```python
from build123d import *

# Parameters (mm, degrees)
SKETCH_1_W                         = 397
SKETCH_1_H                         = 497
SKETCH_1_W_2                       = 22.1
SKETCH_1_H_2                       = 22.1
SM_BASE_FLANGE_1_DEPTH             = 2
SM_EDGE_FLANGE_1_STRIP_W           = 8.6
SM_EDGE_FLANGE_1_STRIP_H           = 2
SM_EDGE_FLANGE_1_STRIP_CUT_DEPTH   = 497
SM_EDGE_FLANGE_1_STRIP_2_W         = 8.6
SM_EDGE_FLANGE_1_STRIP_2_H         = 2
SM_EDGE_FLANGE_1_STRIP_CUT_2_DEPTH = 497
SM_EDGE_FLANGE_1_DEPTH             = 497
SM_EDGE_FLANGE_1_BEND_DEPTH        = 497
SM_START                           = -198.5
SM_EDGE_FLANGE_2_DEPTH             = 397
SM_EDGE_FLANGE_2_2_DEPTH           = 2.3
SM_START_2                         = 196.2
SM_EDGE_FLANGE_2_3_DEPTH           = 2.3
SM_START_3                         = -196.2
SM_EDGE_FLANGE_2_4_DEPTH           = 392.4
SKETCH_18_R                        = 1.6
CUT_EXTRUDE_1_DEPTH                = 10


# Read off the part's stored shape, not the designer's step: 边线-法兰2
# Sheet-metal steps are written as plain solids
with BuildPart() as part:
    # Sketch 1 → 基体-法兰1 (new body)
    with BuildSketch(Plane.XY):
        Rectangle(SKETCH_1_W, SKETCH_1_H)
        with Locations((-146.5, 0)):
            Rectangle(SKETCH_1_W_2, SKETCH_1_H_2, mode=Mode.SUBTRACT)
    extrude(amount=-SM_BASE_FLANGE_1_DEPTH)

    # 边线-法兰1 strip (across the edge) → 边线-法兰1 strip cut (cut)
    with BuildSketch(Plane(origin=(198.5, 248.5, -2), x_dir=(-1, 0, 0), z_dir=(0, -1, 0))):
        with Locations((-2, -1)):
            Rectangle(SM_EDGE_FLANGE_1_STRIP_W, SM_EDGE_FLANGE_1_STRIP_H)
    extrude(amount=SM_EDGE_FLANGE_1_STRIP_CUT_DEPTH, mode=Mode.SUBTRACT)

    # 边线-法兰1 strip 2 (across the edge) → 边线-法兰1 strip cut 2 (cut)
    with BuildSketch(Plane(origin=(-198.5, -248.5, -2), x_dir=(1, 0, 0), z_dir=(0, 1, 0))):
        with Locations((-2, -1)):
            Rectangle(SM_EDGE_FLANGE_1_STRIP_2_W, SM_EDGE_FLANGE_1_STRIP_2_H)
    extrude(amount=SM_EDGE_FLANGE_1_STRIP_CUT_2_DEPTH, mode=Mode.SUBTRACT)

    # 边线-法兰1 section (across the edge) → 边线-法兰1 (add)
    with BuildSketch(Plane(origin=(198.5, 248.5, -2), x_dir=(-1, 0, 0), z_dir=(0, -1, 0))):
        with BuildLine():
            Line((0, 0.3), (0, 13))
            Line((0, 13), (2, 13))
            Line((2, 13), (2, 0.3))
            ThreePointArc((2, 0.3), (2.087867966, 0.087867966), (2.3, 0))
            Line((2.3, 0), (2.3, -2))
            ThreePointArc((2.3, -2), (0.673654403, -1.326345597), (0, 0.3))
        make_face()
    extrude(amount=SM_EDGE_FLANGE_1_DEPTH)

    # 边线-法兰1 section 2 (across the edge) → 边线-法兰1 bend (add)
    with BuildSketch(Plane(origin=(-198.5, -248.5, -2), x_dir=(1, 0, 0), z_dir=(0, 1, 0))):
        with BuildLine():
            Line((0, 0.3), (0, 13))
            Line((0, 13), (2, 13))
            Line((2, 13), (2, 0.3))
            ThreePointArc((2, 0.3), (2.087867966, 0.087867966), (2.3, 0))
            Line((2.3, 0), (2.3, -2))
            ThreePointArc((2.3, -2), (0.673654403, -1.326345597), (0, 0.3))
        make_face()
    extrude(amount=SM_EDGE_FLANGE_1_BEND_DEPTH)

    # 边线-法兰2 outline → 边线-法兰2 (cut)
    with BuildSketch(Plane.YZ.offset(SM_START)):
        with BuildLine():
            Line((-246.5, -2.3), (-246.2, -2.3))
            Line((-246.2, -2.3), (-246.2, -2))
            ThreePointArc((-246.2, -2), (-246.412132034, -2.087867966), (-246.5, -2.3))
        make_face()
        with BuildLine():
            ThreePointArc((-248.5, -2.3), (-247.826345597, -0.673654403), (-246.2, 0))
            Line((-246.2, 0), (-248.5, 0))
            Line((-248.5, 0), (-248.5, -2.3))
        make_face()
        with BuildLine():
            ThreePointArc((246.5, -2.3), (246.412132034, -2.087867966), (246.2, -2))
            Line((246.2, -2), (246.2, -2.3))
            Line((246.2, -2.3), (246.5, -2.3))
        make_face()
        with BuildLine():
            Line((248.5, 0), (246.2, 0))
            ThreePointArc((246.2, 0), (247.826345597, -0.673654403), (248.5, -2.3))
            Line((248.5, -2.3), (248.5, 0))
        make_face()
    extrude(amount=SM_EDGE_FLANGE_2_DEPTH, mode=Mode.SUBTRACT)

    # Sm Edge Flange 2 2 outline → Sm Edge Flange 2 2 (cut)
    with BuildSketch(Plane.YZ.offset(SM_START)):
        with BuildLine():
            Line((-248.5, -2.3), (-246.5, -2.3))
            ThreePointArc((-246.5, -2.3), (-246.412132034, -2.087867966), (-246.2, -2))
            Line((-246.2, -2), (-246.2, 0))
            ThreePointArc((-246.2, 0), (-247.826345597, -0.673654403), (-248.5, -2.3))
        make_face()
        with BuildLine():
            ThreePointArc((248.5, -2.3), (247.826345597, -0.673654403), (246.2, 0))
            Line((246.2, 0), (246.2, -2))
            ThreePointArc((246.2, -2), (246.412132034, -2.087867966), (246.5, -2.3))
            Line((246.5, -2.3), (248.5, -2.3))
        make_face()
    extrude(amount=SM_EDGE_FLANGE_2_2_DEPTH, mode=Mode.SUBTRACT)

    # Sm Edge Flange 2 3 outline → Sm Edge Flange 2 3 (cut)
    with BuildSketch(Plane.YZ.offset(SM_START_2)):
        with BuildLine():
            Line((-248.5, -2.3), (-246.5, -2.3))
            ThreePointArc((-246.5, -2.3), (-246.412132034, -2.087867966), (-246.2, -2))
            Line((-246.2, -2), (-246.2, 0))
            ThreePointArc((-246.2, 0), (-247.826345597, -0.673654403), (-248.5, -2.3))
        make_face()
        with BuildLine():
            ThreePointArc((248.5, -2.3), (247.826345597, -0.673654403), (246.2, 0))
            Line((246.2, 0), (246.2, -2))
            ThreePointArc((246.2, -2), (246.412132034, -2.087867966), (246.5, -2.3))
            Line((246.5, -2.3), (248.5, -2.3))
        make_face()
    extrude(amount=SM_EDGE_FLANGE_2_3_DEPTH, mode=Mode.SUBTRACT)

    # Sm Edge Flange 2 4 outline → Sm Edge Flange 2 4 (add)
    with BuildSketch(Plane.YZ.offset(SM_START_3)):
        with BuildLine():
            Line((-246.5, -15), (-246.5, -2.3))
            ThreePointArc((-246.5, -2.3), (-246.412132034, -2.087867966), (-246.2, -2))
            Line((-246.2, -2), (-248.48035085, -2))
            ThreePointArc((-248.48035085, -2), (-248.495082456, -2.149678603), (-248.5, -2.3))
            Line((-248.5, -2.3), (-248.5, -15))
            Line((-248.5, -15), (-246.5, -15))
        make_face()
        with BuildLine():
            Line((248.48035085, -2), (246.2, -2))
            ThreePointArc((246.2, -2), (246.412132034, -2.087867966), (246.5, -2.3))
            Line((246.5, -2.3), (246.5, -15))
            Line((246.5, -15), (248.5, -15))
            Line((248.5, -15), (248.5, -2.3))
            ThreePointArc((248.5, -2.3), (248.495082456, -2.149678603), (248.48035085, -2))
        make_face()
    extrude(amount=SM_EDGE_FLANGE_2_4_DEPTH)

    # 草图18 → 切除-拉伸1 (cut)
    with BuildSketch(Plane(origin=(198.5, 0, 0), x_dir=(0, 0, -1), z_dir=(1, 0, 0))):
        with Locations((5.5, -183.25)):
            Circle(SKETCH_18_R)
        with Locations((12.5, -183.25)):
            Circle(SKETCH_18_R)
        with Locations((5.5, -168.75)):
            Circle(SKETCH_18_R)
        with Locations((12.5, -168.75)):
            Circle(SKETCH_18_R)
        with Locations(Location((12.5, 168.75, 0), (0, 0, 180))):
            Circle(SKETCH_18_R)
        with Locations(Location((5.5, 168.75, 0), (0, 0, 180))):
            Circle(SKETCH_18_R)
        with Locations(Location((12.5, 183.25, 0), (0, 0, 180))):
            Circle(SKETCH_18_R)
        with Locations(Location((5.5, 183.25, 0), (0, 0, 180))):
            Circle(SKETCH_18_R)
    extrude(amount=-CUT_EXTRUDE_1_DEPTH, mode=Mode.SUBTRACT)


solid = part.part
```
The model under review builds one solid part; all positions refer to its coordinate system, in mm. A direction names the side the tool comes from. Coordinates: 2 decimals unless noted, no trailing zeros. Order: outer loops, then holes, each group sorted by start corner. A loop starts at its lowest first (then second) coordinate and runs counter-clockwise, first axis right, second up. Notation, with made-up numbers: (-35, 35.25) -> (-1, 35.25) arc R26 ccw to (-1, 70.25) -> close; hole circle Ø1 at (-20, 26). An arc over 180 degrees is marked (long way). Answer in a Markdown table with one row per item. Add a question column.
Item 1: We need section B-B on x = -171. Write out the cut boundary in (y, z), plus the area to 3 significant figures.
Item 2: To check wall thickness, follow probe 1 along Y at (x, z) = (197.55, -12.5); probe 2 along Y at (x, z) = (26, -2.25); probe 3 along X at (y, z) = (103.5, -3.5). State the ranges of each line that lie inside material, in increasing order.
Item 3: Machinability: for faces 1 (the flat face through (198.5, 3, -9)), 2 (the flat face through (-3, -246.5, -9)), which of the approach directions +Z, -Z, +X, -X, +Y, -Y give a long, thin tool a straight path to every point of the face, cutting with its end or side? Answer none if there is none.
Item 4: Mouldability with a two-part tool opening along Y and no side actions: class faces 3 (the flat face through (-3, 3, -2)), 4 (the flat face through (-3, 246.5, -9)), 5 (the flat face through (-3, 3, 0)), 6 (the flat face through (-3, -248.5, -9)) as +Y half, -Y half, draft (parallel to the pull), parting line (faces both ways), or undercut.
Item 5: We need section A-A on y = 122.5. Write out the cut boundary in (x, z).
Item 6: Clearance check with flat-ended pins moving along their axes: pin 1 (1 mm diameter, centred on x = 197.5, y = 247, fed in from +Z); pin 2 (2.5 mm diameter, centred on x = 197, z = -1, fed in from +Y); pin 3 (1 mm diameter, centred on x = -141.5, z = -1, fed in from -Y). State where each tip first meets the part, or that it passes through.
Final values:
| question | item | result |
|---|---|---|
| 1 | outline | (-248.5, -15) -> (-246.5, -15) -> (-246.5, -2.3) arc R0.3 cw to (-246.2, -2) -> (246.2, -2) arc R0.3 cw to (246.5, -2.3) -> (246.5, -15) -> (248.5, -15) -> (248.5, -2.3) arc R2.3 ccw to (246.2, 0) -> (-246.2, 0) arc R2.3 ccw to (-248.5, -2.3) -> close |
| 1 | area | 1,040 mm2 |
| 2 | probe 1 | y = -248.5 to -184.85, -181.65 to -170.35, -167.15 to 167.15, 170.35 to 181.65, 184.85 to 248.5 |
| 2 | probe 2 | y = -248.5 to -246.5, 246.5 to 248.5 |
| 2 | probe 3 | x = -198.5 to -196.5, 196.5 to 198.5 |
| 3 | face 1 | +Z, -Z, +X, +Y, -Y |
| 3 | face 2 | -Z |
| 4 | face 3 | undercut |
| 4 | face 4 | undercut |
| 4 | face 5 | draft |
| 4 | face 6 | -Y half |
| 5 | outline | (-198.5, -15) -> (-196.5, -15) -> (-196.5, -2.3) arc R0.3 cw to (-196.2, -2) -> (196.2, -2) arc R0.3 cw to (196.5, -2.3) -> (196.5, -15) -> (198.5, -15) -> (198.5, -2.3) arc R2.3 ccw to (196.2, 0) -> (-196.2, 0) arc R2.3 ccw to (-198.5, -2.3) -> close |
| 6 | pin 1 | stops at z = -2.3 |
| 6 | pin 2 | stops at y = 248.47 |
| 6 | pin 3 | stops at y = -248.36 |
